Build history of the part. All positions in model axes, mm. A direction names the side the tool comes from. Give positions to 0.01 mm unless a question says otherwise; leave off trailing zeros. Write each loop counter-clockwise with the first axis right and the second up, starting at its lowest first coordinate (ties: lowest second). Pieces come first, ordered by that corner, then holes. Notation, with made-up numbers: (36, -10.5) -> (78, -10.5) arc R27 cw to (78, 11.5) -> close; hole circle Ø11 at (81, 38.25). An arc over 180 degrees is marked (long way). One line per question, with ' | ' between items. Start each with the question number.
(1) Pull direction Z, two halves, no side cores. Call faces 1 (the cylindrical face through (5.07, 14.865, -25.77)), 2 (the cylindrical face through (4.93, 14.62, -16.27)), 3 (the cylindrical face through (5.07, 14.88, 25.76)): released by +Z, released by -Z, zero draft, split by the parting line, or undercut.
(2) Tool access for faces 4 (the cylindrical face through (4.93, 22.45, 13.09)), 5 (the cylindrical face through (4.93, -24.78, 8.21)), 6 (the cylindrical face through (4.93, 10.76, 23.79)), 7 (the cylindrical face through (4.93, -10.91, 18.96)): list every direction of +Z, -Z, +X, -X, +Y, -Y with a clear straight run to the whole face (end or side of a thin tool).
(3) Band-saw the part on A-A, the plane z = 0. Give the cut face in (x, y) (3 decimals).
(4) Drill centre lines: probe 1 along Z at (x, y) = (6, 20); probe 2 along Z at (x, y) = (1.5, -27); probe 3 along Y at (x, z) = (2.25, -22). Where is each one in solid material? Low to high. Write a range as from..to.
(5) Band-saw the part on B-B, the plane y = -25.5. Give the cut face in (x, z).
(6) Band-saw the part on C-C, the plane y = -17.5. Give the cut face in (x, z).
(7) Pin check, flat tips, straight feed: P1, Ø1, axis at x = 2.5, y = 4, coming from the -Z side; P2, Ø2, axis at x = 3, y = 17, coming from the -Z side; P3, Ø1, axis at x = 8.5, z = 6.5, coming from the -Y side. Stop position of each tip, or through.
from build123d import *

# Parameters (mm, degrees)
BASPROSKE_W             = 10
BASPROSKE_H             = 29.75
TOOTHCUT_DEPTH          = 44.244941901
TEETHCUTS_COUNT         = 15
TEETHCUTS_ANGLE         = 336
BORSKE_R                = 3.5
BORE_DEPTH              = 50.0000508
SKETCH1_R               = 3.675
CUT_EXTRUDE1_DEPTH      = 10
CUT_EXTRUDE2_DEPTH      = 44.183025
CUT_EXTRUDE2_DEPTH_BACK = 44.183025


with BuildPart() as part:
    # BasProSke → Base-Revolve (revolve)
    with BuildSketch(Plane(origin=(0, 0, 0), x_dir=(1, 0, 0), z_dir=(0, 1, 0)), mode=Mode.PRIVATE) as base_revolve_sk:
        with Locations((5, 14.875)):
            Rectangle(BASPROSKE_W, BASPROSKE_H)
    revolve(base_revolve_sk.sketch.rotate(Axis((-10, 0, 0), (1, 0, 0)), 180), axis=Axis((-10, 0, 0), (1, 0, 0)))

    # TooCutSke → ToothCut (cut, through all)
    with BuildSketch(Plane(origin=(0, 0, 0), x_dir=(0, 0, -1), z_dir=(1, 0, 0))):
        with BuildLine():
            ThreePointArc((1.837264636, 21.796704674), (0, 21.874), (-1.837264636, 21.796704674))
            ThreePointArc((-1.837264636, 21.796704674), (-2.861169083, 25.906231304), (-5.425297323, 29.27696354))
            ThreePointArc((-5.425297323, 29.27696354), (0, 29.7754), (5.425297323, 29.27696354))
            ThreePointArc((5.425297323, 29.27696354), (2.861169083, 25.906231304), (1.837264636, 21.796704674))
        make_face()
    toothcut = extrude(amount=TOOTHCUT_DEPTH, mode=Mode.SUBTRACT)

    # TeethCuts: ToothCut ×15 about axis
    teethcuts_axis = Axis((-10, 0, 0), (1, 0, 0))
    for i in range(1, TEETHCUTS_COUNT):
        add(toothcut.rotate(teethcuts_axis, i * TEETHCUTS_ANGLE / (TEETHCUTS_COUNT - 1)), mode=Mode.SUBTRACT)

    # BorSke → Bore (cut, symmetric)
    with BuildSketch(Plane(origin=(0, 0, 0), x_dir=(0, 0, -1), z_dir=(1, 0, 0))):
        with Locations(Location((0, 0, 0), (0, 0, 180))):
            Circle(BORSKE_R)
    extrude(amount=BORE_DEPTH, both=True, mode=Mode.SUBTRACT)

    # Sketch1 → Cut-Extrude1 (cut)
    with BuildSketch(Plane(origin=(10, 0, 0), x_dir=(0, 0, -1), z_dir=(1, 0, 0))):
        Circle(SKETCH1_R)
    extrude(amount=-CUT_EXTRUDE1_DEPTH, mode=Mode.SUBTRACT)

    # Sketch2 → Cut-Extrude2 (cut, two sides: drawn at the far end of the back side and taken through both)
    with BuildSketch(Plane(origin=(10, 0, 0), x_dir=(0, 0, -1), z_dir=(1, 0, 0)).offset(-CUT_EXTRUDE2_DEPTH_BACK)):
        with BuildLine():
            Line((1.71, 3.252925606), (1.71, 3.675))
            Line((1.71, 3.675), (1.71, 4.175))
            Line((1.71, 4.175), (-1.71, 4.175))
            Line((-1.71, 4.175), (-1.71, 3.675))
            Line((-1.71, 3.675), (-1.71, 3.252925606))
            ThreePointArc((-1.71, 3.252925606), (-0.880659809, 3.567921426), (0, 3.675))
            ThreePointArc((0, 3.675), (0.880659809, 3.567921426), (1.71, 3.252925606))
        make_face()
    extrude(amount=CUT_EXTRUDE2_DEPTH + CUT_EXTRUDE2_DEPTH_BACK, mode=Mode.SUBTRACT)


solid = part.part
Results:
1) face 1: released by -Z | face 2: undercut | face 3: released by +Z
2) face 4: +X, -X, +Y | face 5: +X, -X, -Y | face 6: +Z, +X, -X | face 7: +X, -X
3) outline: (0, -29.75) -> (10, -29.75) -> (10, -3.675) -> (0, -3.675) -> close; (0, 4.175) -> (10, 4.175) -> (10, 21.874) -> (0, 21.874) -> close
4) probe 1: z = -17.54..-11.01, -8.86..8.86, 11.01..17.54 | probe 2: z = -12.49..-10.57, -2.27..2.27, 10.57..12.49 | probe 3: y = -20.03..-17.25, -10.16..-4.19, -0.46..5.16, 9.38..15.42
5) outline: (0, -13.04) -> (10, -13.04) -> (10, -8.83) -> (0, -8.83) -> close; (0, -2.68) -> (10, -2.68) -> (10, 2.68) -> (0, 2.68) -> close; (0, 8.83) -> (10, 8.83) -> (10, 13.04) -> (0, 13.04) -> close
6) outline: (0, -22.1) -> (10, -22.1) -> (10, -15.14) -> (0, -15.14) -> close; (0, -13.12) -> (10, -13.12) -> (10, 13.12) -> (0, 13.12) -> close; (0, 15.14) -> (10, 15.14) -> (10, 22.1) -> (0, 22.1) -> close
7) P1: stops at z = -29.54 | P2: stops at z = -16.6 | P3: stops at y = -22.8
